```python
from build123d import *

# Parameters (mm, degrees)
SKETCH1_R                      = 31.75
SKETCH1_R_2                    = 25.4
SKETCH1_R_3                    = 12.7
SKETCH1_R_4                    = 5
BOSS_EXTRUDE1_DEPTH            = 6.35
F_6_CLEARANCE_HOLE1_AT_2_COUNT = 2
F_6_CLEARANCE_HOLE1_AT_2_PITCH = 19.05
CIRPATTERN1_COUNT              = 4


with BuildPart() as part:
    # Sketch1 → Boss-Extrude1 (new body)
    with BuildSketch(Plane(origin=(0, 0, 0), x_dir=(1, 0, 0), z_dir=(0, 1, 0))):
        Circle(SKETCH1_R)
        Circle(SKETCH1_R_2, mode=Mode.SUBTRACT)
        Circle(SKETCH1_R_3)
        Circle(SKETCH1_R_4, mode=Mode.SUBTRACT)
        with BuildLine():
            ThreePointArc((-12.296722124, -3.175), (-12.7, 0), (-12.296722124, 3.175))
            Line((-12.296722124, 3.175), (-25.200781238, 3.175))
            ThreePointArc((-25.200781238, 3.175), (-25.4, 0), (-25.200781238, -3.175))
            Line((-25.200781238, -3.175), (-12.296722124, -3.175))
        make_face()
        with BuildLine():
            Line((-3.175, 25.200781238), (-3.175, 12.296722124))
            ThreePointArc((-3.175, 12.296722124), (0, 12.7), (3.175, 12.296722124))
            Line((3.175, 12.296722124), (3.175, 25.200781238))
            ThreePointArc((3.175, 25.200781238), (0, 25.4), (-3.175, 25.200781238))
        make_face()
        with BuildLine():
            Line((25.200781238, 3.175), (12.296722124, 3.175))
            ThreePointArc((12.296722124, 3.175), (12.598777143, 1.600254515), (12.7, 0))
            ThreePointArc((12.7, 0), (12.598777143, -1.600254515), (12.296722124, -3.175))
            Line((12.296722124, -3.175), (25.200781238, -3.175))
            ThreePointArc((25.200781238, -3.175), (25.350146385, -1.590621979), (25.4, 0))
            ThreePointArc((25.4, 0), (25.350146385, 1.590621979), (25.200781238, 3.175))
        make_face()
        with BuildLine():
            ThreePointArc((3.175, -12.296722124), (0, -12.7), (-3.175, -12.296722124))
            Line((-3.175, -12.296722124), (-3.175, -25.200781238))
            ThreePointArc((-3.175, -25.200781238), (0, -25.4), (3.175, -25.200781238))
            Line((3.175, -25.200781238), (3.175, -12.296722124))
        make_face()
    extrude(amount=BOSS_EXTRUDE1_DEPTH)

    # Sketch2 → #6 Clearance Hole1 (revolve, cut)
    with BuildSketch(Plane(origin=(0, 6.35, 28.575), x_dir=(0, 0, 1), z_dir=(1, 0, 0))):
        Polygon((0, 0), (0, 13.7988539), (1.8288, 12.7), (1.8288, 0), align=None)
    f_6_clearance_hole1 = revolve(axis=Axis((0, 12.7, 28.575), (0, -1, 0)), mode=Mode.SUBTRACT)

    # #6 Clearance Hole1 at 2: #6 Clearance Hole1 ×2
    with Locations(*[(0, 0, -i * F_6_CLEARANCE_HOLE1_AT_2_PITCH) for i in range(1, F_6_CLEARANCE_HOLE1_AT_2_COUNT)]):
        add(f_6_clearance_hole1, mode=Mode.SUBTRACT)

    # CirPattern1: #6 Clearance Hole1 ×4 about axis
    cirpattern1_axis = Axis((0, 0, 0), (0, 1, 0))
    for i in range(1, CIRPATTERN1_COUNT):
        add(f_6_clearance_hole1.rotate(cirpattern1_axis, i * 360 / CIRPATTERN1_COUNT), mode=Mode.SUBTRACT)

    # CirPattern1 copy 1 sketch → CirPattern1 copy 1 (revolve, cut)
    with BuildSketch(Plane(origin=(9.525, 6.35, 0), x_dir=(1, 0, 0), z_dir=(0, 0, -1))):
        Polygon((0, 0), (0, 13.7988539), (1.8288, 12.7), (1.8288, 0), align=None)
    revolve(axis=Axis((9.525, 12.7, 0), (0, -1, 0)), mode=Mode.SUBTRACT)

    # CirPattern1 copy 2 sketch → CirPattern1 copy 2 (revolve, cut)
    with BuildSketch(Plane(origin=(0, 6.35, -9.525), x_dir=(0, 0, -1), z_dir=(-1, 0, 0))):
        Polygon((0, 0), (0, 13.7988539), (1.8288, 12.7), (1.8288, 0), align=None)
    revolve(axis=Axis((0, 12.7, -9.525), (0, -1, 0)), mode=Mode.SUBTRACT)

    # CirPattern1 copy 3 sketch → CirPattern1 copy 3 (revolve, cut)
    with BuildSketch(Plane(origin=(-9.525, 6.35, 0), x_dir=(-1, 0, 0), z_dir=(0, 0, 1))):
        Polygon((0, 0), (0, 13.7988539), (1.8288, 12.7), (1.8288, 0), align=None)
    revolve(axis=Axis((-9.525, 12.7, 0), (0, -1, 0)), mode=Mode.SUBTRACT)


solid = part.part
```
Verification items for the finished model (mm, model axes). Give positions to 0.01 mm unless a question says otherwise; leave off trailing zeros. Loops run counter-clockwise (first coordinate to the right, second up) from the corner with the lowest first, then second, coordinate; pieces in that order, holes last.
1. Section check C-C, the plane y = 5.25. Count the separate pieces of the cut face and the enclosed holes in it, then the cut area to 3 significant figures.
2. Section check A-A, the plane z = 0. Enter the section's corners in (x, y), then the cut area to 3 significant figures.
3. Mould release check, pull along X, two halves, no side actions. Record for faces 1 (the flat face through (0, 6.35, 7)), 2 (the cylindrical face through (-6.883, 3.131, 30.995)), 3 (the cylindrical face through (0.7, 3.219, 30.264)): released by +X, released by -X, zero draft, split by the parting line, or undercut.
4. Thickness scan on line 1 (Z direction, x = 11, y = 1); line 2 (Z direction, x = -19, y = 1.5) (3 decimals). Record the ranges inside material, lowest first.
5. Section check B-B, the plane x = 0. Enter the section's corners in (y, z), then the cut area to 3 significant figures.
6. Go/stop test with flat-tipped pins: pin 1 Ø1.5 at (x, z) = (5, 23) entering from +Y; pin 2 Ø1.9 at (x, y) = (-18, 2.5) entering from -Z; pin 3 Ø1.9 at (x, y) = (-16.5, 2.5) entering from +Z; pin 4 Ø3 at (x, y) = (18, 3) entering from +Z. Record where each tip stops, or that it passes through.
Geometry says:
1. separate pieces: 1
1. enclosed holes: 13
1. area: 1,810 mm2
2. outline: (-31.75, 0) - (-30.4, 0) - (-30.4, 6.35) - (-31.75, 6.35) - close; (-26.75, 0) - (-11.35, 0) - (-11.35, 6.35) - (-26.75, 6.35) - close; (-7.7, 0) - (-5, 0) - (-5, 6.35) - (-7.7, 6.35) - close; (5, 0) - (7.7, 0) - (7.7, 6.35) - (5, 6.35) - close; (11.35, 0) - (26.75, 0) - (26.75, 6.35) - (11.35, 6.35) - close; (30.4, 0) - (31.75, 0) - (31.75, 6.35) - (30.4, 6.35) - close
2. area: 247 mm2
3. face 1: zero draft
3. face 2: split by the parting line
3. face 3: undercut
4. line 1: z = -29.78 to -22.89, -6.35 to -1.08, 1.08 to 6.35, 22.89 to 29.78
4. line 2: z = -25.437 to -16.857, -3.175 to 3.175, 16.857 to 25.437
5. outline: (0, -31.75) - (6.35, -31.75) - (6.35, -30.4) - (0, -30.4) - close; (0, -26.75) - (6.35, -26.75) - (6.35, -11.35) - (0, -11.35) - close; (0, -7.7) - (6.35, -7.7) - (6.35, -5) - (0, -5) - close; (0, 5) - (6.35, 5) - (6.35, 7.7) - (0, 7.7) - close; (0, 11.35) - (6.35, 11.35) - (6.35, 26.75) - (0, 26.75) - close; (0, 30.4) - (6.35, 30.4) - (6.35, 31.75) - (0, 31.75) - close
5. area: 247 mm2
6. pin 1: passes through
6. pin 2: stops at z = -26.78
6. pin 3: stops at z = 27.68
6. pin 4: stops at z = 27.13
